from build123d import *

# Parameters (mm, degrees)
SKETCH1_R           = 1
SKETCH1_R_2         = 2
BOSS_EXTRUDE1_DEPTH = 4


with BuildPart() as part:
    # Sketch1 → Boss-Extrude1 (new body)
    with BuildSketch(Plane.XY):
        with BuildLine():
            Line((32.768661414, 9.5), (0, 9.5))
            ThreePointArc((0, 9.5), (-5.132216198, 7.994395343), (-8.637676899, 3.954811978))
            ThreePointArc((-8.637676899, 3.954811978), (-13.707021242, -7.117107183), (-1.734430481, -9.340329272))
            ThreePointArc((-1.734430481, -9.340329272), (3.531285703, -8.819298231), (7.70145267, -5.562160262))
            Line((7.70145267, -5.562160262), (18.50145267, -5.562160262))
            Line((18.50145267, -5.562160262), (27.120384516, -8.153301675))
            Line((27.120384516, -8.153301675), (42.092126283, -9.073599712))
            Line((42.092126283, -9.073599712), (44.676644991, -8.438049901))
            Line((44.676644991, -8.438049901), (44.999262596, -8.358716152))
            ThreePointArc((44.999262596, -8.358716152), (52.618268655, -1.863685843), (52.259320622, 8.141604176))
            ThreePointArc((52.259320622, 8.141604176), (50.560022951, 13.41298626), (45.041503714, 13.883121423))
            ThreePointArc((45.041503714, 13.883121423), (38.224286315, 13.597806101), (32.768661414, 9.5))
        make_face()
        with Locations((-8.637676899, -5.562160262)):
            Circle(SKETCH1_R, mode=Mode.SUBTRACT)
        Circle(SKETCH1_R_2, mode=Mode.SUBTRACT)
        with BuildLine():
            ThreePointArc((18.50145267, -2), (16.50145267, 0), (18.50145267, 2))
            Line((18.50145267, 2), (27.120384516, 2))
            ThreePointArc((27.120384516, 2), (29.120384516, 0), (27.120384516, -2))
            Line((27.120384516, -2), (18.50145267, -2))
        make_face(mode=Mode.SUBTRACT)
        with Locations((44.676644991, -3.558553592)):
            Circle(SKETCH1_R_2, mode=Mode.SUBTRACT)
        with Locations((47.447381223, 9.5)):
            Circle(SKETCH1_R, mode=Mode.SUBTRACT)
    extrude(amount=BOSS_EXTRUDE1_DEPTH)


solid = part.part
Could you check a few things on this model? Use its own coordinates, in mm. A direction names the side the tool comes from. Give positions to 0.01 mm unless a question says otherwise; leave off trailing zeros. Order: outer loops, then holes, each group sorted by start corner. A loop starts at its lowest first (then second) coordinate and runs counter-clockwise, first axis right, second up. Notation, with made-up numbers: (27, 25) - (47, 25) arc R21 ccw to (47, 31) - close; hole circle Ø8 at (89, 78). An arc over 180 degrees is marked (long way). Return JSON: item names as keys, results as strings. Group by question number.
Q1. Please list where these lines run through material, in increasing order: line 1 along Y through (x, z) = (18.5, 2.6); line 2 along Y through (x, z) = (19.5, 3.5); line 3 along Y through (x, z) = (15, 2.6). Write a range as [from, to].
Q2. Suppose I cut it at D-D, the plane y = 7. Please give me the cut outline in (x, z), and give its area (3 significant figures).
Q3. Thinking about a two-plate mould opening in Y: for faces 1 (the face through (-13.795, -6.942, 1.972)), 2 (the face through (0, -2, 2)), 3 (the face through (22.75, -6.84, 1.97)), 4 (the face through (19, 5, 0)), which applies, pulls with the +Y half, pulls with the -Y half, needs draft (parallel to the pull), parting line crosses it, or undercut?
Q4. Suppose I cut it at C-C, the plane z = 2.75. Please give me the cut outline in (x, y).
Q5. Will these pins go through, and if not, where does the flat tip stop? pin 1 Ø10 at (x, y) = (0, 1.5) entering from +Z; pin 2 Ø2 at (x, z) = (12.5, 2) entering from +Y; pin 3 Ø1 at (y, z) = (-3, 2) entering from +X; pin 4 Ø1.5 at (y, z) = (11, 1.5) entering from +X.
Q6. Which directions (+Z, -Z, +X, -X, +Y, -Y) give clear straight access to the entire face, cutting with the end or side of a thin tool? Please do faces 5 (the face through (16.5, 0, 2)), 6 (the face through (17, 9.5, 2)), 7 (the face through (34.501, -8.607, 1.972)), 8 (the face through (52.559, -1.996, 1.972)).
Q7. Suppose I cut it at A-A, the plane x = 26. Please give me the cut outline in (y, z).
Q8. Suppose I cut it at B-B, the plane y = 0. Please give me the cut outline in (x, z).
Resolved:
{
 "1": {"line 1": "y = [-5.56, -2], [2, 9.5]", "line 2": "y = [-5.86, -2], [2, 9.5]", "line 3": "y = [-5.56, 9.5]"},
 "2": {"outline": "(-6.42, 0) - (52.79, 0) - (52.79, 4) - (-6.42, 4) - close", "area": "237 mm2"},
 "3": {"face 1": "parting line crosses it", "face 2": "undercut", "face 3": "pulls with the -Y half", "face 4": "needs draft"},
 "4": {"outline": "(-8.64, 3.95) arc R7.72 ccw (long way) to (-1.73, -9.34) arc R9.5 ccw to (7.7, -5.56) - (18.5, -5.56) - (27.12, -8.15) - (42.09, -9.07) - (45, -8.36) arc R11.5 ccw to (52.26, 8.14) arc R5 ccw to (45.04, 13.88) arc R11.5 ccw to (32.77, 9.5) - (0, 9.5) arc R9.5 ccw to start; hole circle Ø2 at (-8.64, -5.56); hole circle Ø4 at (0, 0); hole (18.5, -2) - (27.12, -2) arc R2 ccw to (27.12, 2) - (18.5, 2) arc R2 ccw to start; hole circle Ø4 at (44.68, -3.56); hole circle Ø2 at (47.45, 9.5)"},
 "5": {"pin 1": "stops at z = 4", "pin 2": "stops at y = 9.5", "pin 3": "stops at x = 52.31", "pin 4": "stops at x = 52.39"},
 "6": {"face 5": "+Z, -Z", "face 6": "+Z, -Z, -X, +Y", "face 7": "+Z, -Z, -Y", "face 8": "+Z, -Z, +X"},
 "7": {"outline": "(-7.82, 0) - (-2, 0) - (-2, 4) - (-7.82, 4) - close; (2, 0) - (9.5, 0) - (9.5, 4) - (2, 4) - close"},
 "8": {"outline": "(-13.71, 0) - (-2, 0) - (-2, 4) - (-13.71, 4) - close; (2, 0) - (16.5, 0) - (16.5, 4) - (2, 4) - close; (29.12, 0) - (53.25, 0) - (53.25, 4) - (29.12, 4) - close"}
}
